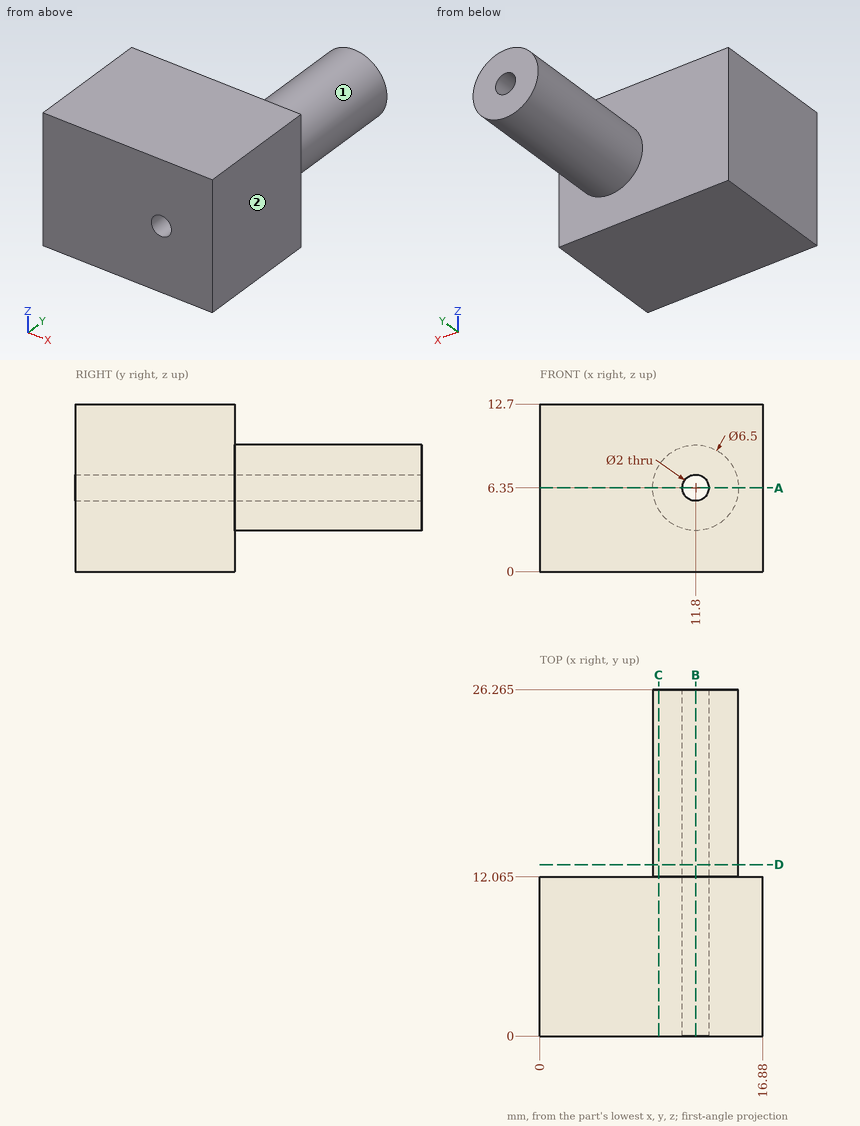
Part print with two shaded views. Sizes in mm from the minimum x, y, z corner. A direction names the side the tool comes from. Round coordinates to 2 decimals unless told otherwise and drop trailing zeros. Write each loop counter-clockwise with the first axis right and the second up, starting at its lowest first coordinate (ties: lowest second). Pieces come first, ordered by that corner, then holes. Notation, with made-up numbers: (-12.75, -28) - (10.25, -28) arc R12 ccw to (10.25, -11) - close; hole circle Ø3 at (-14.5, 53). An arc over 180 degrees is marked (long way). Answer as CSV lines item,"result".
Q1. Cut at D-D (y = 13). Write the cut outline in (x, z), and give its area (3 significant figures).
Report:
outline,"circle Ø6.5 at (11.8, 6.35); hole circle Ø2 at (11.8, 6.35)"
area,"30.0 mm^2"
Q2. Drop flat-ended pins along their axis: pin 1 (8 mm diameter, centred on x = 12.5, y = 16.5, fed in from -Z); pin 2 (3 mm diameter, centred on y = 6.5, z = 2, fed in from -X); pin 3 (6 mm diameter, centred on x = 11, y = 17.5, fed in from +Z); pin 4 (1.5 mm diameter, centred on y = 17, z = 8.5, fed in from +X). Give the stop position or say it passes through.
Report:
pin 1,"stops at z = 3.1"
pin 2,"stops at x = 0"
pin 3,"stops at z = 9.6"
pin 4,"stops at x = 14.73"
Q3. Cut at B-B (x = 11.8). Write the cut outline in (y, z) (3 decimals), and give its area (3 significant figures).
Report:
outline,"(0, 0) - (12.065, 0) - (12.065, 3.1) - (26.265, 3.1) - (26.265, 5.35) - (0, 5.35) - close; (0, 7.35) - (26.265, 7.35) - (26.265, 9.6) - (12.065, 9.6) - (12.065, 12.7) - (0, 12.7) - close"
area,"193 mm^2"
Q4. Drill centre lines: probe 1 along Z at (x, y) = (11.8, 20); probe 2 along X at (y, z) = (7.25, 6.35); probe 3 along X at (y, z) = (19, 6.35). Where is each one in solid material? Low to high. Write a range as [from, to].
Report:
probe 1,"z = [3.1, 5.35], [7.35, 9.6]"
probe 2,"x = [0, 10.8], [12.8, 16.88]"
probe 3,"x = [8.55, 10.8], [12.8, 15.05]"
Q5. Cut at C-C (x = 9). Write the cut outline in (y, z) (3 decimals).
Report:
outline,"(0, 0) - (12.065, 0) - (12.065, 4.7) - (26.265, 4.7) - (26.265, 8) - (12.065, 8) - (12.065, 12.7) - (0, 12.7) - close"
Q6. Cut at A-A (z = 6.35). Write the cut outline in (x, y) (3 decimals), and give its area (3 significant figures).
Report:
outline,"(0, 0) - (10.8, 0) - (10.8, 26.265) - (8.55, 26.265) - (8.55, 12.065) - (0, 12.065) - close; (12.8, 0) - (16.88, 0) - (16.88, 12.065) - (15.05, 12.065) - (15.05, 26.265) - (12.8, 26.265) - close"
area,"243 mm^2"
Q7. Tool access for the marked faces 1 and 2: list every direction of +Z, -Z, +X, -X, +Y, -Y with a clear straight run to the whole face (end or side of a thin tool).
Report:
face 1,"+Y"
face 2,"+Z, -Z, +X, +Y, -Y"
